Geometry: final body of the model. Coordinates: model frame, mm. Give positions to 0.01 mm unless a question says otherwise; leave off trailing zeros. Order: outer loops, then holes, each group sorted by start corner. A loop starts at its lowest first (then second) coordinate and runs counter-clockwise, first axis right, second up. Notation, with made-up numbers: M -8,60.25 L 2,60.25 A10 ccw 2,66.25 Z; hole C 16,47.5 d11. An arc over 180 degrees is marked long. One line per item, written item: value. Start each with the question number.
```python
from build123d import *

# Parameters (mm, degrees)
F0_R     = 10
F1_DEPTH = 1
F2_R     = 20


with BuildPart() as f1:
    # F0 (on Top) → F1 (new body)
    with BuildSketch(Plane.XY):
        with BuildLine():
            Line((0, 0), (-45, 0))
            Line((-45, 0), (-37.5, -50))
            Line((-37.5, -50), (0, -50))
            Line((0, -50), (0, -35))
            ThreePointArc((0, -35), (-10, -25), (0, -15))
            Line((0, -15), (0, 0))
        make_face()
        with Locations((-22, -25)):
            Circle(F0_R, mode=Mode.SUBTRACT)
        with BuildLine():
            Line((45, 0), (0, 0))
            Line((0, 0), (0, -15))
            ThreePointArc((0, -15), (7.071068, -17.928932), (10, -25))
            ThreePointArc((10, -25), (7.071068, -32.071068), (0, -35))
            Line((0, -35), (0, -50))
            Line((0, -50), (37.5, -50))
            Line((37.5, -50), (45, 0))
        make_face()
        with Locations((22, -25)):
            Circle(F0_R, mode=Mode.SUBTRACT)
    extrude(amount=F1_DEPTH)

    # F2
    f2_edges = [f1.edges().sort_by_distance(p)[0] for p in [
        (-37.5, -50, 0.5),
        (37.5, -50, 0.5),
        (45, 0, 0.5),
        (-45, 0, 0.5),
    ]]
    fillet(f2_edges, radius=F2_R)


solid = f1.part
```
Q1. Section query C-C on x = -23. Return loops of the section in (y, z).
Q2. Section query D-D on x = 4. Return loops of the section in (y, z), and give its area (3 significant figures).
Q3. Ray query, line 1 along X through (y, z) = (-24.5, 0.1) (1 decimal); line 2 along Y through (x, z) = (-0.5, 0.2); line 3 along X through (y, z) = (-29, 0.1). Return the intervals inside material, ascending. Write a range as [from, to].
Q4. Section query B-B on z = 0.5. Return loops of the section in (x, y), and give its area (3 significant figures).
Q5. Mould query, pull axis Y, two halves, no side actions, for faces 1 (the face through (9, -19, 1)), 2 (the face through (-12.46, -22, 0.49)), 3 (the face through (40.8, -28, 0.5)). Classes: +Y half, -Y half, draft (parallel to the pull), parting line (faces both ways), or undercut.
Q6. Section query A-A on y = -26.5. Return loops of the section in (x, z) (3 decimals), and give its area (3 significant figures).
Results below:
1. outline: M -49.81,0 L -34.95,0 L -34.95,1 L -49.81,1 Z; M -15.05,0 L -0.04,0 L -0.04,1 L -15.05,1 Z
2. outline: M -50,0 L -34.17,0 L -34.17,1 L -50,1 Z; M -15.83,0 L 0,0 L 0,1 L -15.83,1 Z
2. area: 31.7 mm2
3. line 1: [-41.3, -32], [-12, -10], [10, 12], [32, 41.3]
3. line 2: [-50, -34.99], [-15.01, 0]
3. line 3: [-40.65, -31.17], [-12.83, -9.17], [9.17, 12.83], [31.17, 40.65]
4. outline: M -41.55,-22.97 L -40.05,-32.97 A20 ccw -20.28,-50 L 20.28,-50 A20 ccw 40.05,-32.97 L 41.55,-22.97 A20 ccw 21.78,0 L -21.78,0 A20 ccw Z; hole C -22,-25 d20; hole M 0,-15 A10 ccw long 10,-25 A10 ccw Z; hole C 22,-25 d20
4. area: 2,820 mm2
5. face 1: draft
5. face 2: undercut
5. face 3: -Y half
6. outline: M -41.025,0 L -31.887,0 L -31.887,1 L -41.025,1 Z; M -12.113,0 L -9.887,0 L -9.887,1 L -12.113,1 Z; M 9.887,0 L 12.113,0 L 12.113,1 L 9.887,1 Z; M 31.887,0 L 41.025,0 L 41.025,1 L 31.887,1 Z
6. area: 22.7 mm2
